Source: CAD feature listing. Evaluate the final solid. Frame: model axes, mm. A direction names the side the tool comes from. Coordinates: 2 decimals unless noted, no trailing zeros. Order: outer loops, then holes, each group sorted by start corner. A loop starts at its lowest first (then second) coordinate and runs counter-clockwise, first axis right, second up.
```python
from build123d import *

# Parameters (mm, degrees)
ESQUISSE4_W                  = 18.656759262
ESQUISSE4_H                  = 11.470185
ENL_V_MAT_EXTRU_1_DEPTH      = 10
ENL_V_MAT_EXTRU_1_DEPTH_BACK = 10
ESQUISSE5_R                  = 12.05
ESQUISSE5_R_2                = 11.9
BOSS_EXTRU_1_DEPTH           = 5.6
ESQUISSE6_R                  = 1.5
ENL_V_MAT_EXTRU_2_DEPTH      = 5
R_P_TITION_CIRCULAIRE1_COUNT = 3


with BuildPart() as part:
    # Esquisse1 → R_volution1 (revolve)
    with BuildSketch(Plane.XY):
        Polygon((-30, 0), (-30, 17), (0, 17), (0, 18.4), (22, 18.4), (22, 0), align=None)
    revolve(axis=Axis((-59.117838542, 0, 0), (1, 0, 0)))

    # Esquisse3 → R_volution2 (revolve)
    with BuildSketch(Plane.XY):
        Polygon((22, -1), (28.5, -1), (28.5, -4), (44, -4), (44, -7), (22, -7), align=None)
    revolve(axis=Axis((8.410725031, -7, 0), (1, 0, 0)))

    # Esquisse4 → Enl_v. mat.-Extru.1 (cut, two sides)
    with BuildSketch(Plane.XY) as enl_v_mat_extru_1_sk:
        with Locations((41.328379631, 1.1350925)):
            Rectangle(ESQUISSE4_W, ESQUISSE4_H)
    extrude(amount=ENL_V_MAT_EXTRU_1_DEPTH, mode=Mode.SUBTRACT)
    extrude(enl_v_mat_extru_1_sk.sketch, amount=-ENL_V_MAT_EXTRU_1_DEPTH_BACK, mode=Mode.SUBTRACT)

    # Esquisse5 → Boss.-Extru.1 (add)
    with BuildSketch(Plane.ZY.offset(30)):
        Circle(ESQUISSE5_R)
        Circle(ESQUISSE5_R_2, mode=Mode.SUBTRACT)
    extrude(amount=BOSS_EXTRU_1_DEPTH)

    # Esquisse6 → Enl_v. mat.-Extru.2 (cut)
    with BuildSketch(Plane(origin=(22, 0, 0), x_dir=(0, 0, -1), z_dir=(1, 0, 0))):
        with Locations((0, 15.5)):
            Circle(ESQUISSE6_R)
        with Locations((7.75, 13.423393759)):
            Circle(ESQUISSE6_R)
        with Locations((-7.75, 13.423393759)):
            Circle(ESQUISSE6_R)
    enl_v_mat_extru_2 = extrude(amount=-ENL_V_MAT_EXTRU_2_DEPTH, mode=Mode.SUBTRACT)

    # R_p_tition circulaire1: Enl_v. mat.-Extru.2 ×3 about axis
    r_p_tition_circulaire1_axis = Axis((0, 0, 0), (1, 0, 0))
    for i in range(1, R_P_TITION_CIRCULAIRE1_COUNT):
        add(enl_v_mat_extru_2.rotate(r_p_tition_circulaire1_axis, i * 360 / R_P_TITION_CIRCULAIRE1_COUNT), mode=Mode.SUBTRACT)


solid = part.part
```
1. Ray query, line 1 (Z direction, x = 20, y = -7); line 2 (Y direction, x = 20.55, z = 7.75); line 3 (X direction, y = 4, z = 4.5). Return the intervals inside material, ascending.
Findings:
line 1: z = -17.02 to -14.72, -12.12 to 12.12, 14.72 to 17.02
line 2: y = -16.69 to -14.92, -11.92 to 11.92, 14.92 to 16.69
line 3: x = -30 to 22
2. Access query for faces 5 (the face through (-30, -4, 12)), 6 (the face through (19.535, -14.888, 8.075)). Directions: +Z, -Z, +X, -X, +Y, -Y. A direction counts if a zero-diameter tool reaches every point of the face in a straight line with its end or side. Return the directions, or none.
Findings:
face 5: -X
face 6: +X
3. Section query C-C on x = 33. Return loops of the section in (y, z), plus the area to 3 significant figures.
Findings:
outline: (-4.6, -1.8) - (-4.6, 1.8) arc R3 ccw (long way) to start
area: 26.8 mm2
4. Draft query along Z for faces 1 (the face through (-32.8, 3.6, 11.5)), 2 (the face through (19.54, 11.96, 8.08)), 3 (the face through (-32.761, -7.241, -9.443)), 4 (the face through (38, -4.6, 0)). Return one class per face: released by +Z, released by -Z, zero draft, split by the parting line, or undercut.
Findings:
face 1: split by the parting line
face 2: undercut
face 3: undercut
face 4: zero draft
5. Section query B-B on y = 0. Return loops of the section in (x, z), plus the area to 3 significant figures.
Findings:
outline: (-35.6, -12.05) - (-30, -12.05) - (-30, -17) - (0, -17) - (0, -18.4) - (22, -18.4) - (22, -17) - (17, -17) - (17, -14) - (22, -14) - (22, 14) - (17, 14) - (17, 17) - (22, 17) - (22, 18.4) - (0, 18.4) - (0, 17) - (-30, 17) - (-30, 12.05) - (-35.6, 12.05) - (-35.6, 11.9) - (-30, 11.9) - (-30, -11.9) - (-35.6, -11.9) - close
area: 1,800 mm2
6. Pin query (flat end, axial travel): P1, Ø2.5, axis at y = -7.75, z = -13.42, coming from the +X side; P2, Ø4, axis at x = 13, y = 11, coming from the -Z side; P3, Ø4, axis at x = -24.5, y = 0, coming from the -Z side; P4, Ø11, axis at y = 5.5, z = 3.5, coming from the -X side. Return the tip coordinate at first contact, or that it passes through.
Findings:
P1: stops at x = 17
P2: stops at z = -16.05
P3: stops at z = -17
P4: stops at x = -35.6
